Verification items for the finished model (mm, model axes). Give positions to 0.01 mm unless a question says otherwise; leave off trailing zeros. Loops run counter-clockwise (first coordinate to the right, second up) from the corner with the lowest first, then second, coordinate; pieces in that order, holes last. Notation, with made-up numbers: M 22.25,60 L 79.25,60 A34 cw 79.25,98 Z; hole C -11.75,-24.5 d4. An arc over 180 degrees is marked long. Use CSV: the item, a comma, the result in double quotes.
from build123d import *

# Parameters (mm, degrees)
BOSS_EXTRUDE1_START = 1
SKETCH1_R           = 1.4
BOSS_EXTRUDE1_DEPTH = 32
SKETCH2_R           = 2.35
BOSS_EXTRUDE2_DEPTH = 3
FILLET1_R           = 2
BOSS_EXTRUDE3_START = 3
SKETCH3_R           = 2.35
BOSS_EXTRUDE3_DEPTH = 3
FILLET2_R           = 2


with BuildPart() as part:
    # Sketch1 → Boss-Extrude1 (new body)
    with BuildSketch(Plane(origin=(15, 0, 0), x_dir=(0, 0, -1), z_dir=(1, 0, 0)).offset(BOSS_EXTRUDE1_START)):
        with Locations((32.233241632, 33)):
            Circle(SKETCH1_R)
    extrude(amount=-BOSS_EXTRUDE1_DEPTH)

    # Sketch2 → Boss-Extrude2 (add)
    with BuildSketch(Plane(origin=(16, 0, 0), x_dir=(0, 0, -1), z_dir=(1, 0, 0))):
        with Locations((32.233241632, 33)):
            Circle(SKETCH2_R)
    extrude(amount=BOSS_EXTRUDE2_DEPTH)

    # Fillet1
    # the kernel refuses this fillet: 2 mm, written as the material it adds along each edge
    with BuildSketch(Plane(origin=(16, 33, -32.233241632), x_dir=(0, 0, -1), z_dir=(0, -1, 0))) as fillet1_piece_1:
        with BuildLine():
            CenterArc((3.4, -1.702204453), FILLET1_R, 121.668243254, 58.331756746)
            Line((1.4, -1.702204453), (1.4, 0))
            Line((1.4, 0), (2.35, 0))
        make_face()
    revolve(axis=Axis((16, 33, -32.233241632), (1, 0, 0)))
    # the kernel refuses this fillet: 2 mm, written as the material it takes off along each edge
    with BuildSketch(Plane(origin=(19, 33, -32.233241632), x_dir=(0, 0, -1), z_dir=(0, -1, 0))) as fillet1_2_piece_1:
        with BuildLine():
            CenterArc((2.35 - FILLET1_R, -FILLET1_R), FILLET1_R, 0, 90)
            Line((2.35 - FILLET1_R, 0), (2.35, 0))
            Line((2.35, 0), (2.35, -FILLET1_R))
        make_face()
    revolve(axis=Axis((19, 33, -32.233241632), (1, 0, 0)), mode=Mode.SUBTRACT)

    # Sketch3 → Boss-Extrude3 (add)
    with BuildSketch(Plane.ZY.offset(16).offset(BOSS_EXTRUDE3_START)):
        with Locations(Location((-32.233241632, 33, 0), (0, 0, 180))):
            Circle(SKETCH3_R)
    extrude(amount=-BOSS_EXTRUDE3_DEPTH)

    # Fillet2
    # the kernel refuses this fillet: 2 mm, written as the material it adds along each edge
    with BuildSketch(Plane(origin=(-16, 33, -32.233241632), x_dir=(0, 0, -1), z_dir=(0, -1, 0))) as fillet2_piece_1:
        with BuildLine():
            CenterArc((3.4, 1.702204453), FILLET2_R, 180, 58.331756746)
            Line((1.4, 1.702204453), (1.4, 0))
            Line((1.4, 0), (2.35, 0))
        make_face()
    revolve(axis=Axis((-16, 33, -32.233241632), (1, 0, 0)))
    # the kernel refuses this fillet: 2 mm, written as the material it takes off along each edge
    with BuildSketch(Plane(origin=(-19, 33, -32.233241632), x_dir=(0, 0, -1), z_dir=(0, 1, 0))) as fillet2_2_piece_1:
        with BuildLine():
            CenterArc((2.35 - FILLET2_R, -FILLET2_R), FILLET2_R, 360, 90)
            Line((2.35 - FILLET2_R, 0), (2.35, 0))
            Line((2.35, 0), (2.35, -FILLET2_R))
        make_face()
    revolve(axis=Axis((-19, 33, -32.233241632), (-1, 0, 0)), mode=Mode.SUBTRACT)


solid = part.part
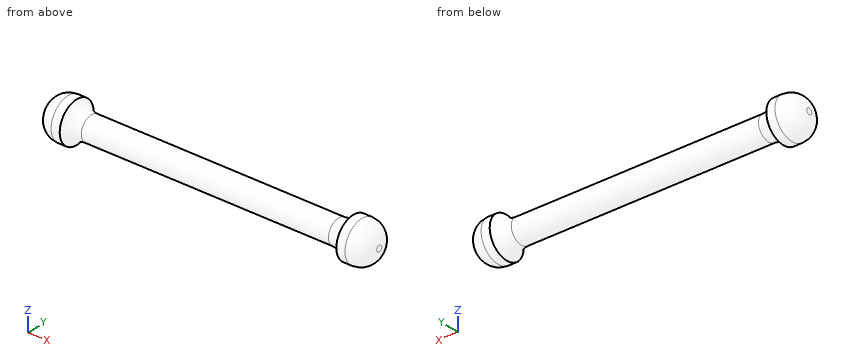
(1) Scan lines: L1, parallel to Z at x = -6.5, y = 33.1; L2, parallel to Y at x = 7, z = -32.25; L3, parallel to X at y = 31.25, z = -31.8. Record each from-to range of solid material in increasing order. Write a range as from..to.
Calculated:
L1,"z = -33.63..-30.84"
L2,"y = 31.6..34.4"
L3,"x = -18.37..-15.5, 15.5..18.37"
(2) Depth check by flat-ended pin: pin 1 Ø1 at (x, y) = (13.5, 31.5) entering from +Z; pin 2 Ø2 at (y, z) = (31.5, -32.5) entering from +X; pin 3 Ø1 at (y, z) = (34.5, -34) entering from -X. Enter the tip coordinate at first touch or a pass-through.
Calculated:
pin 1,"stops at z = -31.25"
pin 2,"stops at x = 18.99"
pin 3,"stops at x = -18.36"
(3) Section check A-A on x = 9.5. Record the cut outline in (y, z), plus the area to 3 significant figures.
Calculated:
outline,"C 33,-32.23 d2.8"
area,"6.16 mm²"
